Read the model definition and answer for the solid it produces. Units are mm, in the model's axes. Face numbers are marked on the shaded views. A direction names the side the tool comes from. Coordinates: 2 decimals unless noted, no trailing zeros. Loops run counter-clockwise (first coordinate to the right, second up) from the corner with the lowest first, then second, coordinate; pieces in that order, holes last. Notation, with made-up numbers: (49, -16) -> (81, -16) arc R27 ccw to (81, 9) -> close; hole circle Ø1 at (52, -21.5). An arc over 180 degrees is marked (long way). One line per question, with ' | ' between items. Start each with the question number.
```python
from build123d import *

# Parameters (mm, degrees)
F1_DEPTH = 2
F2_DEPTH = 1
F0_W     = 20.5
F0_H     = 84
F3_DEPTH = 37.5


with BuildPart() as f1:
    # F0 (on Top) → F1 (new body)
    with BuildSketch(Plane.XY):
        with BuildLine():
            Line((-51.746925, 15), (84.753075, 15))
            Line((84.753075, 15), (100.597961, 26.64865))
            Line((100.597961, 26.64865), (100.597961, 33.64865))
            Line((100.597961, 33.64865), (80.097961, 33.64865))
            Line((80.097961, 33.64865), (80.097961, 117.64865))
            Line((80.097961, 117.64865), (100.597961, 117.64865))
            Line((100.597961, 117.64865), (100.597961, 129.14865))
            ThreePointArc((100.597961, 129.14865), (89.497411, 135.405037), (85.097961, 147.363693))
            Line((85.097961, 147.363693), (85.097961, 211.818904))
            ThreePointArc((85.097961, 211.818904), (89.538305, 223.443985), (100.597961, 229.14865))
            Line((100.597961, 229.14865), (100.597961, 237.548321))
            Line((100.597961, 237.548321), (79.1298, 237.548321))
            Line((79.1298, 237.548321), (79.1298, 265))
            Line((79.1298, 265), (-48.949795, 265))
            Line((-48.949795, 265), (-48.949795, 237.548321))
            Line((-48.949795, 237.548321), (-63.902039, 237.548321))
            Line((-63.902039, 237.548321), (-63.902039, 180.590159))
            Line((-63.902039, 180.590159), (-63.902039, 117.64865))
            Line((-63.902039, 117.64865), (-43.402039, 117.64865))
            Line((-43.402039, 117.64865), (-43.402039, 33.64865))
            Line((-43.402039, 33.64865), (-63.902039, 33.64865))
            Line((-63.902039, 33.64865), (-63.902039, 26.64865))
            Line((-63.902039, 26.64865), (-51.746925, 15))
        make_face()
    extrude(amount=F1_DEPTH)

    # F0 (on Top) → F2 (join)
    with BuildSketch(Plane.XY):
        with BuildLine():
            ThreePointArc((85.097961, 147.363693), (89.497411, 135.405037), (100.597961, 129.14865))
            Line((100.597961, 129.14865), (100.597961, 229.14865))
            ThreePointArc((100.597961, 229.14865), (89.538305, 223.443985), (85.097961, 211.818904))
            Line((85.097961, 211.818904), (85.097961, 147.363693))
        make_face()
        Polygon((-51.746925, 0), (0, 0), (84.753075, 0), (84.753075, 15), (-51.746925, 15), align=None)
    extrude(amount=F2_DEPTH)

    # F0 (on Top) → F3 (join)
    with BuildSketch(Plane.XY):
        with Locations((90.347961, 75.64865)):
            Rectangle(F0_W, F0_H)
        with Locations((-53.652039, 75.64865)):
            Rectangle(F0_W, F0_H)
    extrude(amount=F3_DEPTH)


solid = f1.part
```
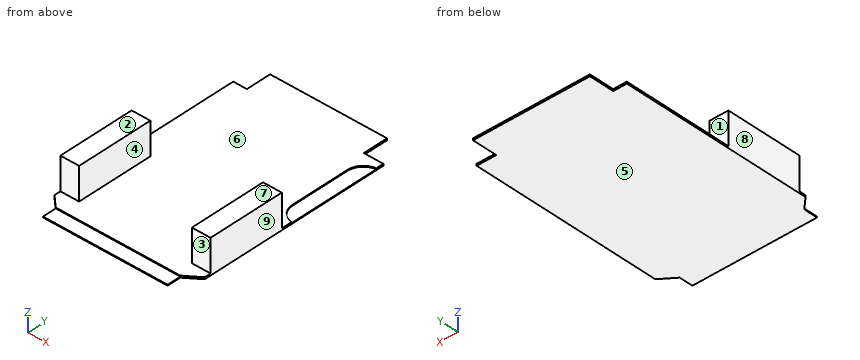
(1) Section A-A on z = 6.5 is taken. Write down the section's boundary in (x, y).
(2) Find the intervals of material crossed by probe 1 along X at (y, z) = (71.5, 10.5); probe 2 along Z at (x, y) = (68, 243.5); probe 3 along Y at (x, z) = (-53, 29), in increasing order. Write a range as from..to.
(3) Section D-D on y = 204 is taken. Write down the section's boundary in (x, z).
(4) Each of these flat-tipped pins is pushed along its axis until it touches: pin 1 Ø10 at (x, z) = (91.5, 12.5) entering from -Y; pin 2 Ø2 at (y, z) = (248, 1) entering from -X; pin 3 Ø16.5 at (x, y) = (-2, 7) entering from +Z. Where does it stop, or does it pass through?
(5) Section C-C on y = 63 is taken. Write down the section's boundary in (x, z).
(6) Determine the mould class of the marked faces 6, 7, 8 and 9 for opening direction X: +X half, -X half, draft (parallel to the pull), parting line (faces both ways), or undercut.
(7) Section B-B on x = -22.5 is taken. Write down the section's boundary in (y, z), plus the area to 3 significant figures.
(8) A tool of negligible diameter and unlimited length cuts with its end or side. For the marked faces 1, 2, 3, 4 and 5, from which of +Z, -Z, +X, -X, +Y, -Y can it reach the whole face along a straight path? Write none if from no direction.
Working result:
1) outline: (-63.9, 33.65) -> (-43.4, 33.65) -> (-43.4, 117.65) -> (-63.9, 117.65) -> close; (80.1, 33.65) -> (100.6, 33.65) -> (100.6, 117.65) -> (80.1, 117.65) -> close
2) probe 1: x = -63.9..-43.4, 80.1..100.6 | probe 2: z = 0..2 | probe 3: y = 33.65..117.65
3) outline: (-63.9, 0) -> (100.6, 0) -> (100.6, 1) -> (85.1, 1) -> (85.1, 2) -> (-63.9, 2) -> close
4) pin 1: stops at y = 33.65 | pin 2: stops at x = -48.95 | pin 3: stops at z = 2
5) outline: (-63.9, 0) -> (100.6, 0) -> (100.6, 37.5) -> (80.1, 37.5) -> (80.1, 2) -> (-43.4, 2) -> (-43.4, 37.5) -> (-63.9, 37.5) -> close
6) face 6: undercut | face 7: draft | face 8: -X half | face 9: +X half
7) outline: (0, 0) -> (265, 0) -> (265, 2) -> (15, 2) -> (15, 1) -> (0, 1) -> close | area: 515 mm2
8) face 1: +Z, +X, -X, +Y | face 2: +Z, +X, -X, +Y, -Y | face 3: +Z, +X, -X, -Y | face 4: +Z, +Y, -Y | face 5: -Z, +X, -X, +Y, -Y
